Geometry: final body of the model. Coordinates: model frame, mm. A direction names the side the tool comes from. Give positions to 0.01 mm unless a question says otherwise; leave off trailing zeros. Write each loop counter-clockwise with the first axis right and the second up, starting at its lowest first coordinate (ties: lowest second). Pieces come first, ordered by that corner, then holes.
Autodesk Inventor part; units mm, degrees
ref_plane "YZ Plane" through (0, 0, 0) normal (1, 0, 0) x (0, 1, 0)
ref_plane "XZ Plane" through (0, 0, 0) normal (0, 1, 0) x (-1, 0, 0)
ref_plane "XY Plane" through (0, 0, 0) normal (0, 0, 1) x (1, 0, 0)
sketch "Sketch1" plane through (0, 0, 0) normal (0, 1, 0) x (-1, 0, 0)
  line L0 (1.7184, 7.0425) -> (-7.8416, 7.0425)
  line L1 (-7.8416, -8.1575) -> (1.7184, -8.1575)
  line L2 (1.7184, -8.1575) -> (1.7184, 7.0425)
  circle A0 centre (-3.2816, 5.5425) radius 1.15
  circle A1 centre (-3.2816, -6.6575) radius 1.15
  line L3 (-7.8416, 7.0425) -> (-7.8416, 3.5425)
  line L4 (-7.8416, -4.6575) -> (-7.8416, -8.1575)
  arc A2 (-7.8416, -4.6575) -> (-7.8416, 3.5425) centre (-7.8416, -0.5575) ccw
  point P0 (0, 0)
  dimension "d0" = 15.2
  dimension "d2" = 5
  dimension "d3" = 5
  dimension "d4" = 1.5
  dimension "d5" = 1.5
  dimension "d6" = 2.3
  dimension "d7" = 2.3
  dimension "d11" = 9.56
  dimension "d12" = 8.2
  dimension "d13" = 7.6
extrude "Extrusion1" add sketch "Sketch1" along normal blind 6
sketch "Sketch2" plane through (0, 6, 0) normal (0, 1, 0) x (1, 0, 0)
  line L0 (-1.7184, -7.0425) -> (7.8416, -7.0425)
  line L1 (-1.7184, 8.1575) -> (-1.7184, -7.0425)
  line L2 (7.8416, -7.0425) -> (-1.7184, -7.0425)
  line L3 (-1.7184, -7.0425) -> (-1.7184, -3.3925)
  line L4 (-1.7184, -3.3925) -> (7.8416, -3.3925)
  line L5 (7.8416, -3.3925) -> (7.8416, -7.0425)
  line L6 (7.8416, 4.5075) -> (-1.7184, 4.5075)
  line L7 (-1.7184, 4.5075) -> (-1.7184, 8.1575)
  line L8 (-1.7184, 8.1575) -> (7.8416, 8.1575)
  line L9 (7.8416, 8.1575) -> (7.8416, 4.5075)
  point P0 (0, 0)
  dimension "d14" = 3.65
  dimension "d19" = 3.65
extrude "Extrusion2" cut sketch "Sketch2" against normal blind 4 contours L1 L4 L5 L0
extrude "Extrusion3" cut sketch "Sketch2" against normal blind 4 contours L1 L8 L9 L6
properties part number "UCover_SMA"
Q1. Section B-B on y = 0.85. Output: boundary loops of the cut face in (x, z), plus the area to 3 significant figures.
Filled sheet:
outline: (-1.72, -8.16) - (7.84, -8.16) - (7.84, -4.66) arc R4.1 cw to (7.84, 3.54) - (7.84, 7.04) - (-1.72, 7.04) - close; hole circle Ø2.3 at (3.28, -6.66); hole circle Ø2.3 at (3.28, 5.54)
area: 111 mm2
Q2. Section C-C on x = 6. Output: boundary loops of the cut face in (y, z), plus the area to 3 significant figures.
Filled sheet:
outline: (0, -8.16) - (2, -8.16) - (2, -4.51) - (6, -4.51) - (6, -4.22) - (0, -4.22) - close; (0, 3.11) - (6, 3.11) - (6, 3.39) - (2, 3.39) - (2, 7.04) - (0, 7.04) - close
area: 18.0 mm2
Q3. Access query for faces 1 (the flat face through (3, 4, -4.508)), 2 (the flat face through (7.842, 1, 5)), 3 (the flat face through (2, 4, 3.392)). Directions: +Z, -Z, +X, -X, +Y, -Y. A direction counts if a zero-diameter tool reaches every point of the face in a straight line with its end or side. Return the directions, or none.
Filled sheet:
face 1: -Z, +X, -X, +Y
face 2: +Z, -Z, +X, +Y, -Y
face 3: +Z, +X, -X, +Y
Q4. Section A-A on x = 0.75. Output: boundary loops of the cut face in (y, z), plus the area to 3 significant figures.
Filled sheet:
outline: (0, -8.16) - (2, -8.16) - (2, -4.51) - (6, -4.51) - (6, 3.39) - (2, 3.39) - (2, 7.04) - (0, 7.04) - close
area: 62.0 mm2
Q5. Ray query, line 1 along X through (y, z) = (1.1, -6.75); line 2 along Y through (x, z) = (1, -5.75); line 3 along X through (y, z) = (1.8, -0.75). Return the intervals inside material, ascending.
Filled sheet:
line 1: x = -1.72 to 2.14, 4.43 to 7.84
line 2: y = 0 to 2
line 3: x = -1.72 to 3.75
Q6. Pull-direction query (X, two-part tool) for faces 4 (the flat face through (7.842, 1, -6)), 5 (the cylindrical face through (4.194, 0.986, -5.958)), 6 (the flat face through (2, 6, -1)); classes: released by +X, released by -X, zero draft, split by the parting line, or undercut.
Filled sheet:
face 4: released by +X
face 5: undercut
face 6: zero draft
Q7. Pin query (flat end, axial travel): P1, Ø1, axis at x = 4.5, y = 4, coming from the -Z side; P2, Ø1.8, axis at x = 3.28, z = -6.66, coming from the -Y side; P3, Ø1.8, axis at x = 1.5, z = -6, coming from the +Y side; P4, Ø1.2, axis at x = 2.5, y = 3.5, coming from the +Z side. Return the tip coordinate at first contact, or that it passes through.
Filled sheet:
P1: stops at z = -4.51
P2: passes through
P3: stops at y = 2
P4: stops at z = 3.39
Q8. Section D-D on z = -6.5. Output: boundary loops of the cut face in (x, y), plus the area to 3 significant figures.
Filled sheet:
outline: (-1.72, 0) - (2.14, 0) - (2.14, 2) - (-1.72, 2) - close; (4.42, 0) - (7.84, 0) - (7.84, 2) - (4.42, 2) - close
area: 14.6 mm2
